Geometry check sheet. Reference: the model listing, model coordinates, mm. A direction names the side the tool comes from. Round coordinates to 2 decimals unless told otherwise and drop trailing zeros. Order: outer loops, then holes, each group sorted by start corner. A loop starts at its lowest first (then second) coordinate and runs counter-clockwise, first axis right, second up. Notation, with made-up numbers: (61.5, -33) - (104.5, -33) arc R4 ccw to (104.5, -28) - close; hole circle Ø7 at (88.5, 38). An arc over 180 degrees is marked (long way). Use a Markdown table: item, result. Add a question column.
(1) Access from +Z, -Z, +X, -X, +Y, -Y to the whole of each face (thin tool, end or side, straight path). Record for faces 1 (the face through (0, 39, 0)), 2 (the face through (11.16, -11.47, 55.14)), 3 (the face through (-27, -28, 50)), 4 (the face through (30.61, -7.98, 27.26)), 5 (the face through (3, 43, 10)).
(2) Gauge pin test, flat ends, axial feed: P1, Ø12, axis at y = -41, z = 46.5, coming from the -X side; P2, Ø4, axis at x = -8.5, y = -40, coming from the -Z side; P3, Ø4, axis at y = 43, z = 20, coming from the -X side. Record the tip position at first contact, or that the pin passes through.
(3) Section check D-D on y = 20.5. Record the boundary of the cut face in (x, z).
(4) Mould release check, pull along Y, two halves, no side actions. Record for faces 6 (the face through (30.834, 8.206, 27.255)), 7 (the face through (-39, 0, 0)), 8 (the face through (34.32, -0.2, 5.07)), 9 (the face through (-19, -19, 45)): released by +Y, released by -Y, zero draft, split by the parting line, or undercut.
(5) Thickness scan on line 1 along Z through (x, y) = (-33.5, 4); line 2 along X through (y, z) = (-39, 5); line 3 along X through (y, z) = (5, 24). Record the ranges inside material, lowest first. Write a range as [from, to].
(6) Section check C-C on x = 18. Record the boundary of the cut face in (y, z), then the cut area to 3 significant figures.
(7) Section check B-B on z = 59. Record the boundary of the cut face in (x, y).
(8) Section check A-A on z = 28. Record the boundary of the cut face in (x, y).
```python
from build123d import *

# Parameters (mm, degrees)
BOSS_EXTRU_1_DEPTH        = 50
BOSS_EXTRU_1_DEPTH_BACK   = 5
BOSS_EXTRU_1_2_DEPTH      = 50
BOSS_EXTRU_1_2_DEPTH_BACK = 5
BOSS_EXTRU_1_3_DEPTH      = 50
BOSS_EXTRU_1_3_DEPTH_BACK = 5
BOSS_EXTRU_1_4_DEPTH      = 50
BOSS_EXTRU_1_4_DEPTH_BACK = 5
BOSS_EXTRU_2_DEPTH        = 20
ESQUISSE4_R               = 4.5
BOSS_EXTRU_3_DEPTH        = 10


with BuildPart() as part:
    # Esquisse1 → Boss.-Extru.1 (new, two sides: drawn at the far end of the back side and taken through both)
    with BuildSketch(Plane.XY.offset(15).offset(-BOSS_EXTRU_1_DEPTH_BACK)):
        Polygon((0, 55), (-16.186291501, 38.813708499), (0, 22.627416998), (16.186291501, 38.813708499), align=None)
    extrude(amount=BOSS_EXTRU_1_DEPTH + BOSS_EXTRU_1_DEPTH_BACK)



with BuildPart() as body_2:
    # Esquisse1 → Boss.-Extru.1 2 (new, two sides: drawn at the far end of the back side and taken through both)
    with BuildSketch(Plane.XY.offset(15).offset(-BOSS_EXTRU_1_2_DEPTH_BACK)):
        Polygon((-38.813708499, 16.186291501), (-55, 0), (-38.813708499, -16.186291501), (-22.627416998, 0), align=None)
    extrude(amount=BOSS_EXTRU_1_2_DEPTH + BOSS_EXTRU_1_2_DEPTH_BACK)


with BuildPart() as body_3:
    # Esquisse1 → Boss.-Extru.1 3 (new, two sides: drawn at the far end of the back side and taken through both)
    with BuildSketch(Plane.XY.offset(15).offset(-BOSS_EXTRU_1_3_DEPTH_BACK)):
        Polygon((-16.186291501, -38.813708499), (0, -55), (16.186291501, -38.813708499), (0, -22.627416998), align=None)
    extrude(amount=BOSS_EXTRU_1_3_DEPTH + BOSS_EXTRU_1_3_DEPTH_BACK)


with BuildPart() as body_4:
    # Esquisse1 → Boss.-Extru.1 4 (new, two sides: drawn at the far end of the back side and taken through both)
    with BuildSketch(Plane.XY.offset(15).offset(-BOSS_EXTRU_1_4_DEPTH_BACK)):
        Polygon((38.813708499, -16.186291501), (55, 0), (38.813708499, 16.186291501), (22.627416998, 0), align=None)
    extrude(amount=BOSS_EXTRU_1_4_DEPTH + BOSS_EXTRU_1_4_DEPTH_BACK)


with BuildPart() as part_1:
    add(part.part)

    add(body_2.part)  # Boss.-Extru.2 merges body 2

    add(body_3.part)  # Boss.-Extru.2 merges body 3

    add(body_4.part)  # Boss.-Extru.2 merges body 4
    # Esquisse3 → Boss.-Extru.2 (add)
    with BuildSketch(Plane.XY.offset(65)):
        Polygon((22.627416998, 0), (0, 22.627416998), (16.186291501, 38.813708499), (38.813708499, 16.186291501), align=None)
        Polygon((-38.813708499, 16.186291501), (-16.186291501, 38.813708499), (0, 22.627416998), (-22.627416998, 0), align=None)
        Polygon((38.813708499, -16.186291501), (16.186291501, -38.813708499), (0, -22.627416998), (22.627416998, 0), align=None)
        Polygon((-38.813708499, -16.186291501), (-22.627416998, 0), (0, -22.627416998), (-16.186291501, -38.813708499), align=None)
    extrude(amount=-BOSS_EXTRU_2_DEPTH)

    # Esquisse4 → Boss.-Extru.3 (add)
    with BuildSketch(Plane(origin=(0, 0, 10), x_dir=(-1, 0, 0), z_dir=(0, 0, -1))):
        with Locations(Location((0, -38.813708499, 0), (0, 0, 180))):
            Circle(ESQUISSE4_R)
        with Locations(Location((-38.813708499, 0, 0), (0, 0, 180))):
            Circle(ESQUISSE4_R)
        with Locations(Location((0, 38.813708499, 0), (0, 0, 180))):
            Circle(ESQUISSE4_R)
        with Locations(Location((38.813708499, 0, 0), (0, 0, 180))):
            Circle(ESQUISSE4_R)
    extrude(amount=BOSS_EXTRU_3_DEPTH)


solid = part_1.part
```
Check sheet entries:
| question | item | result |
|---|---|---|
| 1 | face 1 | -Z, +X, -X, +Y, -Y |
| 1 | face 2 | +Z, -Z |
| 1 | face 3 | +Z, -Z, -X, -Y |
| 1 | face 4 | -Z, -Y |
| 1 | face 5 | -Z |
| 2 | P1 | stops at x = -20 |
| 2 | P2 | stops at z = 10 |
| 2 | P3 | stops at x = -14 |
| 3 | outline | (-34.5, 45) - (-2.13, 45) - (-2.13, 65) - (-34.5, 65) - close; (2.13, 45) - (34.5, 45) - (34.5, 65) - (2.13, 65) - close |
| 4 | face 6 | released by +Y |
| 4 | face 7 | zero draft |
| 4 | face 8 | split by the parting line |
| 4 | face 9 | undercut |
| 5 | line 1 | z = [10, 65] |
| 5 | line 2 | x = [-4.5, 4.5] |
| 5 | line 3 | x = [-50, -27.63], [27.63, 50] |
| 6 | outline | (-37, 45) - (-4.63, 45) - (-4.63, 65) - (-37, 65) - close; (4.63, 45) - (37, 45) - (37, 65) - (4.63, 65) - close |
| 6 | area | 1,290 mm2 |
| 7 | outline | (-55, 0) - (0, -55) - (55, 0) - (0, 55) - close; hole (-22.63, 0) - (0, -22.63) - (22.63, 0) - (0, 22.63) - close |
| 8 | outline | (-55, 0) - (-38.81, -16.19) - (-22.63, 0) - (-38.81, 16.19) - close; (-16.19, -38.81) - (0, -55) - (16.19, -38.81) - (0, -22.63) - close; (-16.19, 38.81) - (0, 22.63) - (16.19, 38.81) - (0, 55) - close; (22.63, 0) - (38.81, -16.19) - (55, 0) - (38.81, 16.19) - close |
